Can you work these out from the drawing? Everything is in mm from the part's minimum corner. A direction names the side the tool comes from. Coordinates: 2 decimals unless noted, no trailing zeros. Order: outer loops, then holes, each group sorted by start corner. A loop starts at its lowest first (then second) coordinate and runs counter-clockwise, first axis right, second up. Notation, with made-up numbers: (50.25, 39.25) -> (62.25, 39.25) arc R15 ccw to (62.25, 45.25) -> close; hole circle Ø11 at (36, 3.25). An arc over 180 degrees is marked (long way). Use a Markdown table: item, result. Add a question column.
1) Thinking about a two-plate mould opening in Z: for the marked faces 3, 4 and 5, which applies, +Z half, -Z half, draft (parallel to the pull), parting line (faces both ways), or undercut?
2) If I drill on L1, parallel to Z at x = 15, y = 7.8; L2, parallel to X at y = 2.5, z = 17.75; L3, parallel to Y at x = 13.75, z = 15.25, over which ranges is the centre line in solid material (lowest first)? Write a range as [from, to].
3) If we section it at A-A (x = 3.75): Write out the boundary of the cut face in (y, z), plus the area to 3 significant figures.
4) Will these pins go through, and if not, where does the flat tip stop? pin 1 Ø0.9 at (y, z) = (2.5, 17) entering from -X; pin 2 Ø7 at (x, y) = (12.5, 19) entering from +Z.
5) If we section it at C-C (z = 14.25): Write out the boundary of the cut face in (x, y), plus the area to 3 significant figures.
6) If we section it at D-D (y = 19): Write out the boundary of the cut face in (x, z).
7) If we section it at B-B (y = 7.8): Write out the boundary of the cut face in (x, z), plus the area to 4 significant figures.
8) Which directions (+Z, -Z, +X, -X, +Y, -Y) give clear straight access to the entire face, cutting with the end or side of a thin tool? Please do the marked faces 1 and 2.
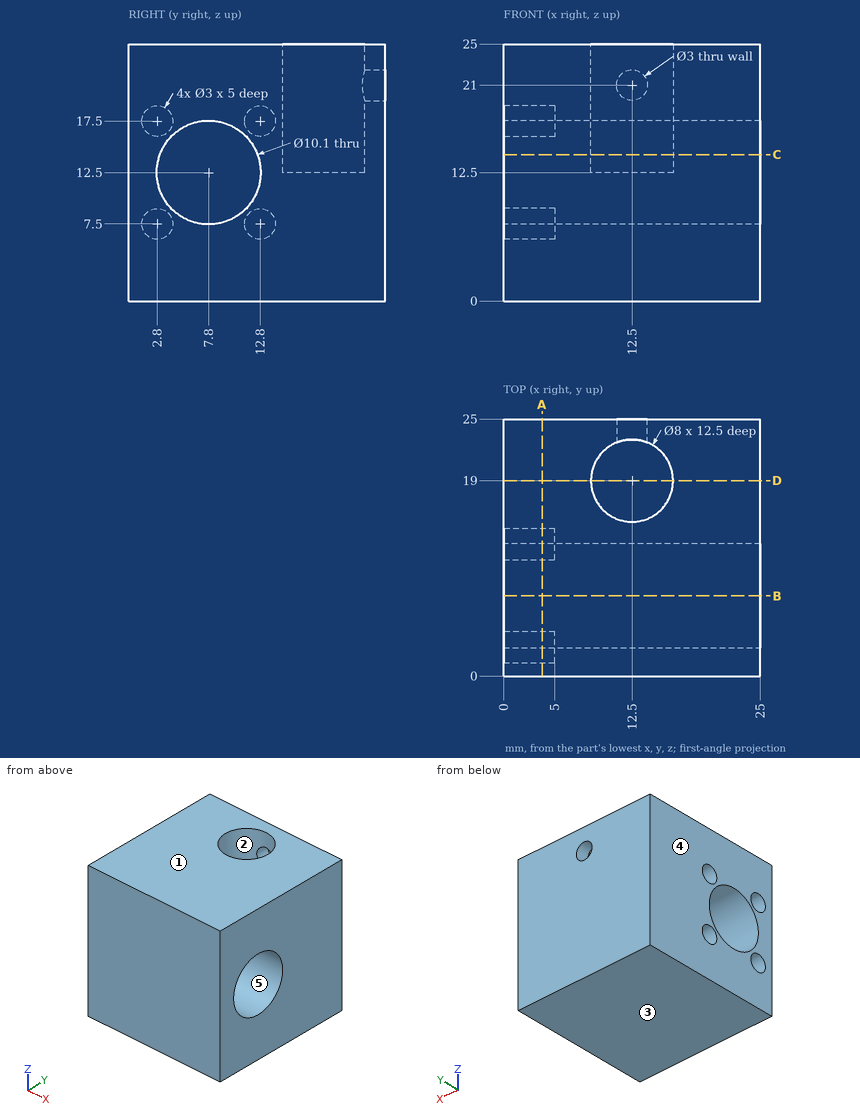
Answer sheet:
| question | item | result |
|---|---|---|
| 1 | face 3 | -Z half |
| 1 | face 4 | draft |
| 1 | face 5 | undercut |
| 2 | L1 | [0, 7.45], [17.55, 25] |
| 2 | L2 | [5, 25] |
| 2 | L3 | [0, 3.56], [12.04, 15.2], [22.8, 25] |
| 3 | outline | (0, 0) -> (25, 0) -> (25, 25) -> (0, 25) -> close; hole circle Ø3 at (2.8, 7.5); hole circle Ø3 at (2.8, 17.5); hole circle Ø10.1 at (7.8, 12.5); hole circle Ø3 at (12.8, 7.5); hole circle Ø3 at (12.8, 17.5) |
| 3 | area | 517 mm2 |
| 4 | pin 1 | x = 5 |
| 4 | pin 2 | z = 12.5 |
| 5 | outline | (0, 0) -> (25, 0) -> (25, 3.06) -> (0, 3.06) -> close; (0, 12.54) -> (25, 12.54) -> (25, 25) -> (0, 25) -> close; hole circle Ø8 at (12.5, 19) |
| 5 | area | 338 mm2 |
| 6 | outline | (0, 0) -> (25, 0) -> (25, 25) -> (16.5, 25) -> (16.5, 12.5) -> (8.5, 12.5) -> (8.5, 25) -> (0, 25) -> close |
| 7 | outline | (0, 0) -> (25, 0) -> (25, 7.45) -> (0, 7.45) -> close; (0, 17.55) -> (25, 17.55) -> (25, 25) -> (0, 25) -> close |
| 7 | area | 372.5 mm2 |
| 8 | face 1 | +Z, +X, -X, +Y, -Y |
| 8 | face 2 | +Z |
